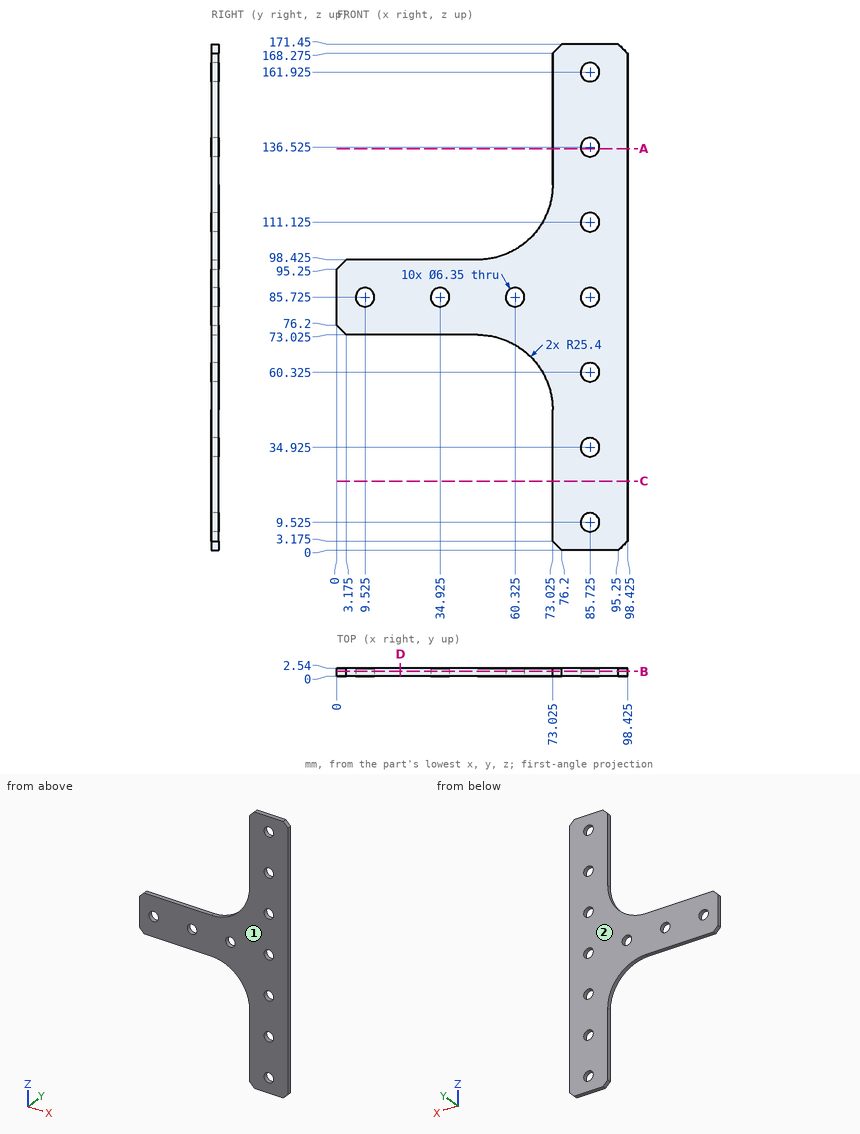
Verification items for this drawing (mm, ordinates from the low corner). Coordinates: 2 decimals unless noted, no trailing zeros. Order: outer loops, then holes, each group sorted by start corner. A loop starts at its lowest first (then second) coordinate and runs counter-clockwise, first axis right, second up. Notation, with made-up numbers: M 68,8 L 101,8 A11 ccw 101,14 Z; hole C -20.5,73 d3. An arc over 180 degrees is marked long. Write each question's results on one line, items separated by ' | '.
1) Scan lines: line 1 along X through (y, z) = (0.35, 162) (3 decimals); line 2 along Z through (x, y) = (16.5, 1.85) (3 decimals). Record each from-to range of solid material in increasing order. Write a range as [from, to].
Solved:
line 1: x = [73.025, 82.551], [88.899, 98.425] | line 2: z = [73.025, 98.425]
2) Release check for a two-part mould opening along Y. For the marked faces 1 and 2 record: pulls with the +Y half, pulls with the -Y half, needs draft (parallel to the pull), parting line crosses it, or undercut.
Solved:
face 1: pulls with the -Y half | face 2: pulls with the +Y half
3) Gauge pin test, flat ends, axial feed: pin 1 Ø1.5 at (x, y) = (74, 0.5) entering from -Z; pin 2 Ø0.8 at (y, z) = (2, 151) entering from -X (3 decimals). Record the tip position at first contact, or that the pin passes through.
Solved:
pin 1: stops at z = 1.45 | pin 2: stops at x = 73.025
4) Section check A-A on z = 136. Record the cut outline in (x, y) (3 decimals), plus the area to 3 significant figures.
Solved:
outline: M 73.025,0 L 82.594,0 L 82.594,2.54 L 73.025,2.54 Z; M 88.856,0 L 98.425,0 L 98.425,2.54 L 88.856,2.54 Z | area: 48.6 mm²
5) Section check D-D on x = 21.5. Record the cut outline in (y, z) (3 decimals), plus the area to 3 significant figures.
Solved:
outline: M 0,73.025 L 2.54,73.025 L 2.54,98.425 L 0,98.425 Z | area: 64.5 mm²
6) Section check C-C on z = 23.5. Record the cut outline in (x, y) (3 decimals).
Solved:
outline: M 73.025,0 L 98.425,0 L 98.425,2.54 L 73.025,2.54 Z
7) Section check B-B on y = 1.55. Give the number of separate pieces and of enclosed holes in the cut face, plus the area to 3 significant figures.
Solved:
separate pieces: 1 | enclosed holes: 10 | area: 6,140 mm²
